Verification items for the finished model (mm, model axes). Face numbers are marked on the shaded views. A direction names the side the tool comes from. Give positions to 0.01 mm unless a question says otherwise; leave off trailing zeros. Write each loop counter-clockwise with the first axis right and the second up, starting at its lowest first coordinate (ties: lowest second). Pieces come first, ordered by that corner, then holes. Notation, with made-up numbers: M 48,43.5 L 67,43.5 A22 cw 67,52.5 Z; hole C 81,-22 d2. An arc over 180 degrees is marked long. Answer as a JSON object with one key per item and string values.
Autodesk Inventor part; units mm, degrees
ref_plane "Work Plane2" through (-35.5643, -7, -23.7485) normal (0, -1, 0) x (0.7068322, 0, -0.7073813)
ref_plane "YZ Plane" through (0, 0, 0) normal (1, 0, 0) x (0, 1, 0)
ref_plane "XZ Plane" through (0, 0, 0) normal (0, 1, 0) x (-1, 0, 0)
ref_plane "Work Plane1" through (-20.7895, 15.2, 8.1501) normal (-0.3618889, 0, -0.9322212) x (-0.9322212, 0, 0.3618889)
sketch "Sketch2" plane through (-20.7895, 15.2, 8.1501) normal (-0.3618889, 0, -0.9322212) x (-0.9322212, 0, 0.3618889)
  circle A0 centre (-11, 0) radius 1
  circle A1 centre (0, 11) radius 1
  circle A2 centre (0, -11) radius 1
  circle A3 centre (-11, 0) radius 3
  circle A4 centre (0, 11) radius 3
  circle A5 centre (0, -11) radius 3
  line L0 (0, 11) -> (3, 11)
  line L1 (0, -11) -> (3, -11)
  line L2 (3, -11) -> (3, 11)
  line L3 (0, 11) -> (-2.1213, 13.1213)
  line L4 (-2.1213, 13.1213) -> (-13.1213, 2.1213)
  line L5 (-13.1213, 2.1213) -> (-11, 0)
  line L6 (3, -11) -> (3, -14)
  line L7 (3, -14) -> (-14, -14)
  line L8 (-14, -14) -> (-14, 0)
  point P0 (-22.3298, -15.2)
  dimension "d6" = 6
  dimension "d4" = 6
  dimension "d5" = 6
  dimension "d7" = 3
extrude "Extrusion1" add sketch "Sketch2" along normal blind 3 contours A0 | L0 L3 A1 | L0 A4 L3 A1 | A1 L3 L0 | A1 L3 A4 L0 | L2 A5 L7 L8 A3 L4 A4 | A5 | L6 L7 A5 | A3 | A2
sketch "Sketch4" plane through (-23.5861, 1.2, 9.2357) normal (0, -1, 0) x (0.9322212, 0, -0.3618889)
  line L0 (25.9951, -3.0341) -> (28.4579, -2.8567)
  line L1 (27.3233, 0.0694) -> (28.4579, -2.8567)
  line L2 (27.3233, 0.0694) -> (25.3298, -0.0742)
  line L3 (25.3298, -0.0742) -> (6.5565, -7.362)
  line L4 (6.5565, -7.362) -> (-4.0222, -15.9035)
  line L5 (-2.8836, -18.8399) -> (-4.0222, -15.9035)
  line L6 (-2.8836, -18.8399) -> (8.0776, -9.9896)
  line L7 (8.0776, -9.9896) -> (25.9951, -3.0341)
  line L8 (17, 0) -> (0, 0)
  line L9 (0, 0) -> (0, -3)
  line L10 (17, -3) -> (0, -3)
  line L11 (17, 0) -> (17, -3)
  line L12 (6.5565, -7.362) -> (6.5565, 0)
  line L13 (17, 0) -> (0, 0)
  line L14 (25.3298, -0.0742) -> (24.2441, 2.7225)
  line L15 (24.2441, 2.7225) -> (17.2311, 0)
  line L16 (17, 0) -> (17, -3)
  line L17 (17, 0) -> (17.2311, 0)
  point P0 (6.5565, 0)
  dimension "d11" = 3
ref_plane "Work Plane2" through (-35.5643, -7, -23.7485) normal (0, -1, 0) x (0.7068322, 0, -0.7073813)
extrude "Extrusion2" add sketch "Sketch4" along normal up to surface (8.2 mm away) contours L3 L12 L10 L11 L17 L15 L14 | L12 L8 L11 L10
sketch "Sketch5" plane through (-23.5861, 1.2, 9.2357) normal (0, 1, 0) x (0.9322212, 0, -0.3618889)
  line L0 (17, 0) -> (17, 3)
  line L1 (17.2311, 0) -> (17, 0)
  line L2 (24.2441, -2.7225) -> (17.2311, 0)
  line L3 (25.3298, 0.0742) -> (24.2441, -2.7225)
  line L4 (6.5565, 7.362) -> (25.3298, 0.0742)
  line L5 (6.5565, 3) -> (6.5565, 7.362)
  line L6 (17, 3) -> (6.5565, 3)
  line L7 (24.2441, -2.7225) -> (17.2311, 0)
  line L8 (24.2441, -2.7225) -> (24.2139, -2.8004)
  line L9 (24.2139, -2.8004) -> (17, 0)
  point P0 (25.3298, 0.0742)
extrude "Extrusion3" add sketch "Sketch5" against normal up to surface (8.2 mm away) contours L1 L2 L8 L9
sketch "Sketch6" plane through (-24.6718, 1.2, 6.4391) normal (0, -1, 0) x (0.9322212, 0, -0.3618889)
  line L0 (6.5565, 0) -> (6.5565, 3)
  line L1 (6.5565, 3) -> (0, 3)
  line L2 (0, 3) -> (0, 0)
  line L3 (6.5565, 0) -> (0, 0)
  line L4 (6.5565, -4.362) -> (6.5565, 3)
  line L5 (6.5565, 0) -> (0, 0)
  line L6 (6.5565, 0) -> (6.5565, -4.362)
  line L7 (0, 0) -> (6.5565, -4.362)
  point P0 (25.3298, 2.9258)
extrude "Extrusion4" add sketch "Sketch6" along normal up to surface (8.2 mm away)
sketch "Sketch7" plane through (0, -7, 0) normal (0, 0, -1) x (-1, 0, 0)
  circle A0 centre (3.0691, 4) radius 1.6
  circle A1 centre (17.0691, 4) radius 1.6
  circle A2 centre (3.0691, 4) radius 1.6
  line L0 (20.1383, 8) -> (0, 8)
  line L1 (20.1383, 8) -> (20.1383, 0)
  line L2 (0, 0) -> (20.1383, 0)
  line L3 (0, 8) -> (0, 0)
  circle A3 centre (3.0691, 4) radius 1
  circle A4 centre (17.0691, 4) radius 1
  point P0 (0, 7)
  dimension "d21" = 2
  dimension "d22" = 2
extrude "Extrusion5" cut sketch "Sketch7" against normal blind 10 contours A3 | A4
ref_plane "Work Plane3" through (-7.7384, 1.2, 3.0836) normal (0, 0, 1) x (1, 0, 0)
sketch "Sketch8" plane through (-7.7384, 1.2, 3.0836) normal (0, 0, 1) x (1, 0, 0)
  circle A0 centre (-9.3308, -4.2) radius 1
  line L0 (-9.3308, -4.2) -> (-9.3308, -11.2) construction
  line L1 (-11.8308, -4.2) -> (-11.8308, -11.2)
  line L2 (-6.8308, -11.2) -> (-6.8308, -4.2)
  arc A1 (-6.8308, -4.2) -> (-11.8308, -4.2) centre (-9.3308, -4.2) ccw
  arc A2 (-11.8308, -11.2) -> (-6.8308, -11.2) centre (-9.3308, -11.2) ccw
  point P0 (7.7384, -1.2)
  point P1 (-9.3308, -7.7)
  dimension "d26" = 7
  dimension "d27" = 5
extrude "Extrusion6" cut sketch "Sketch8" along normal blind 10
sketch "Sketch9" plane through (-21.8751, 15.2, 5.3534) normal (-0.3618889, 0, -0.9322212) x (-0.9322212, 0, 0.3618889)
  circle A0 centre (-11, 0) radius 1
  circle A1 centre (0, 11) radius 1
  circle A2 centre (0, -11) radius 1
  circle A3 centre (0, -11) radius 1
  circle A4 centre (-11, 0) radius 1
  circle A5 centre (0, 11) radius 1
  point P0 (-22.3298, -15.2)
  dimension "d30" = 2
  dimension "d31" = 2
  dimension "d32" = 2
extrude "Extrusion7" cut sketch "Sketch9" against normal blind 10
thicken "Thicken1" operation add thickness 0.2 both sides no extend neighbours yes toward (0, -1, 0) faces at (-17.878, 1.2, 2.242)
sketch "Sketch13" plane through (-21.8751, 15.2, 5.3534) normal (-0.3618889, 0, -0.9322212) x (-0.9322212, 0, 0.3618889)
  line L0 (3, -14.2) -> (3, 11)
  arc A0 (3, 11) -> (-2.1213, 13.1213) centre (0, 11) ccw
  line L1 (-2.1213, 13.1213) -> (-13.1213, 2.1213)
  arc A1 (-13.1213, 2.1213) -> (-14, 0) centre (-11, 0) ccw
  line L2 (-14, 0) -> (-14, -14.2)
  line L3 (-14, -14.2) -> (3, -14.2)
  circle A2 centre (-11, 0) radius 1
  circle A3 centre (0, 11) radius 1
  circle A4 centre (0, -11) radius 1
  line L4 (0, -11) -> (-10, -11)
  line L5 (-11, 0) -> (-21, 0)
  line L6 (0, 11) -> (-10, 11)
  circle A5 centre (-21, 0) radius 3
  circle A6 centre (-10, -11) radius 3
  circle A7 centre (-10, 11) radius 3
  line L7 (-10, 11) -> (-10, 14)
  circle A8 centre (0, 11) radius 1
  line L8 (0, 11) -> (0, 14)
  arc A9 (3, 11) -> (-2.1213, 13.1213) centre (0, 11) ccw
  line L9 (0, 14) -> (-10, 14)
  line L10 (-10, 11) -> (-12.1213, 13.1213)
  line L11 (-21, 0) -> (-23.1213, 2.1213)
  line L12 (-23.1213, 2.1213) -> (-12.1213, 13.1213)
  line L13 (-21, 0) -> (-24, 0)
  line L14 (-3.5565, -14.2) -> (-22.3298, -14.2)
  line L15 (-24, 0) -> (-24, -14.2)
  line L16 (-22.3298, -14.2) -> (-24, -14.2)
  point P0 (-22.3298, -15.2)
  dimension "d57" = 10
  dimension "d58" = 10
  dimension "d59" = 10
  dimension "d60" = 6
  dimension "d61" = 6
  dimension "d62" = 6
extrude "Extrusion11" add sketch "Sketch13" against normal up to surface (3 mm away) contours A0 L1 L6 A7 L9 | L14 L16 L15 A5 L5 L2 | L7 L10 A7 | A7 L6 L7 | L5 A5 L12 A7 L6 L1 A1 | A7 L10 L6 | A5 L13 L5 | L5 L11 A5 | L11 L13 A5
sketch "Sketch14" plane through (-21.8751, 15.2, 5.3534) normal (-0.3618889, 0, -0.9322212) x (-0.9322212, 0, 0.3618889)
  line L0 (3, -14.2) -> (3, 11)
  arc A0 (3, 11) -> (0, 14) centre (0, 11) ccw
  line L1 (0, 14) -> (-10, 14)
  arc A1 (-10, 14) -> (-12.1213, 13.1213) centre (-10, 11) ccw
  line L2 (-12.1213, 13.1213) -> (-23.1213, 2.1213)
  arc A2 (-23.1213, 2.1213) -> (-24, 0) centre (-21, 0) ccw
  line L3 (-24, 0) -> (-24, -14.2)
  line L4 (-24, -14.2) -> (-14.793, -14.2)
  line L5 (3, -14.2) -> (-14.793, -14.2)
  circle A3 centre (-11, 0) radius 1
  circle A4 centre (0, 11) radius 1
  circle A5 centre (0, -11) radius 1
  circle A6 centre (-21, 0) radius 1
  circle A7 centre (0, -11) radius 1
  line L6 (0, -11) -> (-10, -11)
  circle A8 centre (-10, -11) radius 1
  circle A9 centre (0, 11) radius 1
  line L7 (0, 11) -> (-10, 11)
  circle A10 centre (-10, 11) radius 1
  point P0 (-22.3298, -15.2)
  dimension "d65" = 2
  dimension "d66" = 10
  dimension "d67" = 2
  dimension "d68" = 10
  dimension "d69" = 2
extrude "Extrusion12" cut sketch "Sketch14" against normal blind 4 contours A6 | A8 | A10
sketch "Sketch15" plane through (-21.8751, 15.2, 5.3534) normal (-0.3618889, 0, -0.9322212) x (-0.9322212, 0, 0.3618889)
  circle A0 centre (-10, 11) radius 1
  circle A1 centre (-10, -11) radius 1
  circle A2 centre (-21, 0) radius 1
  line L0 (3, -14.2) -> (3, 11)
  arc A3 (3, 11) -> (0, 14) centre (0, 11) ccw
  line L1 (0, 14) -> (-10, 14)
  arc A4 (-10, 14) -> (-12.1213, 13.1213) centre (-10, 11) ccw
  line L2 (-12.1213, 13.1213) -> (-23.1213, 2.1213)
  arc A5 (-23.1213, 2.1213) -> (-24, 0) centre (-21, 0) ccw
  line L3 (-24, 0) -> (-24, -14.2)
  line L4 (-24, -14.2) -> (-14.793, -14.2)
  line L5 (3, -14.2) -> (-14.793, -14.2)
  circle A6 centre (-11, 0) radius 1
  circle A7 centre (0, 11) radius 1
  circle A8 centre (0, -11) radius 1
  point P0 (-22.3298, -15.2)
extrude "Extrusion13" add sketch "Sketch15" against normal up to surface (3 mm away) contours A6 | A7 | A8
sketch "Sketch16" plane through (-21.8751, 15.2, 5.3534) normal (-0.3618889, 0, -0.9322212) x (-0.9322212, 0, 0.3618889)
  circle A0 centre (-10, 11) radius 1
  circle A1 centre (-10, -11) radius 1
  circle A2 centre (-21, 0) radius 1
  line L0 (3, -14.2) -> (3, 11)
  arc A3 (3, 11) -> (0, 14) centre (0, 11) ccw
  line L1 (0, 14) -> (-10, 14)
  arc A4 (-10, 14) -> (-12.1213, 13.1213) centre (-10, 11) ccw
  line L2 (-12.1213, 13.1213) -> (-23.1213, 2.1213)
  arc A5 (-23.1213, 2.1213) -> (-24, 0) centre (-21, 0) ccw
  line L3 (-24, 0) -> (-24, -14.2)
  line L4 (-24, -14.2) -> (-14.793, -14.2)
  line L5 (3, -14.2) -> (-14.793, -14.2)
  circle A6 centre (-10, 11) radius 3
  circle A7 centre (-10, 11) radius 1
  line L6 (-10, 11) -> (-7, 11)
  line L7 (-7, 11) -> (-7, -14.2)
  line L8 (3, -14.2) -> (-14.793, -14.2)
  point P0 (-22.3298, -15.2)
  point P1 (-10, 14)
  dimension "d74" = 6
extrude "Extrusion14" cut sketch "Sketch16" against normal blind 4 contours L5 L7 A6 L1 A3 L0
properties part number "jc_conn_1"
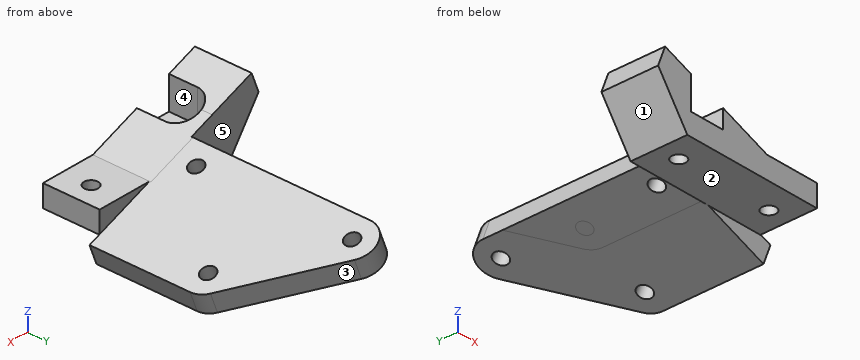
1) Thickness scan on L1, parallel to Y at x = -1, z = 2; L2, parallel to Y at x = -3.75, z = 0.75; L3, parallel to X at y = -5, z = 6.5. Record the ranges inside material, lowest first.
Completed:
{"L1": "y = -7 to 1", "L2": "y = -7 to -3.73, -2.27 to 21.88", "L3": "x = -24.65 to -19.57"}
2) Go/stop test with flat-tipped pins: pin 1 (3.5 mm diameter, centred on x = -5.5, z = 1, fed in from +Y); pin 2 (5 mm diameter, centred on y = 17, z = 0.5, fed in from -X); pin 3 (6 mm diameter, centred on y = -1.5, z = 3.5, fed in from +X). Record where each tip stops, or that it passes through.
Completed:
{"pin 1": "stops at y = 25.35", "pin 2": "stops at x = -15.35", "pin 3": "stops at x = 0"}
3) Section check C-C on x = -12. Count the separate pieces of the cut face and the enclosed holes in it, and give its area (3 significant figures).
Completed:
{"separate pieces": "3", "enclosed holes": "0", "area": "116 mm2"}
4) Access from +Z, -Z, +X, -X, +Y, -Y to the whole of each face (thin tool, end or side, straight path). Record for the marked faces 1 and 2.
Completed:
{"face 1": "-Z, -X, +Y, -Y", "face 2": "-Z, +X, -X, -Y"}
5) Release check for a two-part mould opening along X. For the marked faces 3, 4 and 5 record: pulls with the +X half, pulls with the -X half, needs draft (parallel to the pull), parting line crosses it, or undercut.
Completed:
{"face 3": "pulls with the +X half", "face 4": "undercut", "face 5": "needs draft"}
6) Section check B-B on x = -5.75. Record the boundary of the cut face in (y, z).
Completed:
{"outline": "M -7,0 L 1,0 L 1,-0.91 L 23.15,-0.91 L 24.31,2.31 L 1,2.31 L 1,3.08 L -7,3.08 Z"}
7) Section check A-A on y = 2. Record the boundary of the cut face in (x, z), and give its area (3 significant figures).
Completed:
{"outline": "M -15.35,2.82 L 0.5,-3.33 L 1.58,-0.54 L -14.26,5.62 Z", "area": "51.0 mm2"}
